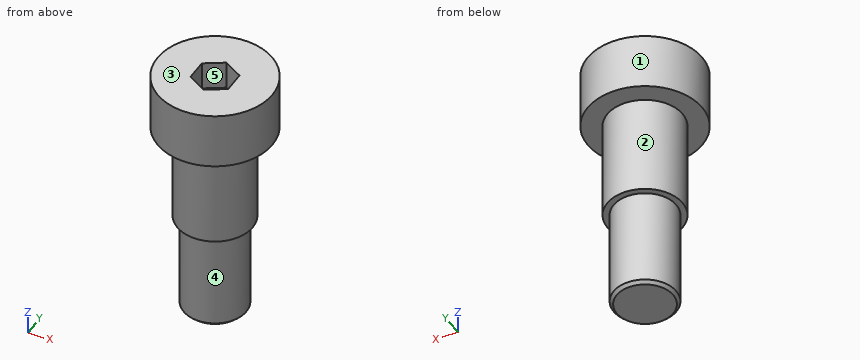
Solid Edge part; units mm, degrees
sketch "Sketch1" plane through (0, 0, 0) normal (0, 0, 1) x (1, 0, 0)
  circle A0 centre (0, 0) radius 9.135
extrude "Protrusion1" add sketch "Sketch1" along normal blind 9
sketch "Sketch2" plane through (0, 0, 9) normal (0, 0, 1) x (1, 0, 0)
  line L0 (0, -3.4641) -> (-3, -1.7321)
  line L1 (-3, -1.7321) -> (-3, 1.7321)
  line L2 (-3, 1.7321) -> (0, 3.4641)
  line L3 (0, 3.4641) -> (3, 1.7321)
  line L4 (3, 1.7321) -> (3, -1.7321)
  line L5 (3, -1.7321) -> (0, -3.4641)
extrude "Cutout1" cut sketch "Sketch2" against normal blind 4.5
sketch "Sketch3" plane through (0, 0, 0) normal (0, 0, -1) x (0, 1, 0)
  circle A0 centre (0, 0) radius 6
extrude "Protrusion2" add sketch "Sketch3" along normal blind 16
sketch "Sketch4" plane through (0, 0, -16) normal (0, 0, -1) x (0, 1, 0)
  circle A0 centre (0, 0) radius 5
extrude "Protrusion3" add sketch "Sketch4" along normal blind 16
chamfer "Chamfer1" distance 0.5 angle 45 1 edges at (0, -5, -32)
properties part number "221437"
Work out the finished part from the listing and answer in its coordinate system (mm). Face numbers are marked on the shaded views. A direction names the side the tool comes from. Round coordinates to 2 decimals unless told otherwise and drop trailing zeros. Loops run counter-clockwise (first coordinate to the right, second up) from the corner with the lowest first, then second, coordinate; pieces in that order, holes last.
(1) The mould has two halves that part along Y. Classify the marked faces 3, 4 and 5: pulls with the +Y half, pulls with the -Y half, needs draft (parallel to the pull), parting line crosses it, or undercut.
Computed values:
face 3: needs draft
face 4: parting line crosses it
face 5: undercut
(2) The part is cut by section B-B, the plane x = -5.5. Give the vertices of the cut face in (y, z).
Computed values:
outline: (-7.29, 0) - (-2.4, 0) - (-2.4, -16) - (2.4, -16) - (2.4, 0) - (7.29, 0) - (7.29, 9) - (-7.29, 9) - close
(3) The part is cut by section A-A, the plane y = 0. Give the vertices of the cut face in (x, z) (3 decimals).
Computed values:
outline: (-9.135, 0) - (-6, 0) - (-6, -16) - (-5, -16) - (-5, -31.5) - (-4.5, -32) - (4.5, -32) - (5, -31.5) - (5, -16) - (6, -16) - (6, 0) - (9.135, 0) - (9.135, 9) - (3, 9) - (3, 4.5) - (-3, 4.5) - (-3, 9) - (-9.135, 9) - close
(4) Find the intervals of material crossed by L1, parallel to Z at x = 3.75, y = 6.5; L2, parallel to Z at x = -0.25, y = -2.75; L3, parallel to X at y = -1.5, z = 5, in increasing order.
Computed values:
L1: z = 0 to 9
L2: z = -32 to 4.5
L3: x = -9.01 to -3, 3 to 9.01
(5) The part is cut by section C-C, the plane z = -15. Give the vertices of the cut face in (x, y), and give its area (3 significant figures).
Computed values:
outline: circle Ø12 at (0, 0)
area: 113 mm2
(6) The part is cut by section D-D, the plane z = 1. Give the vertices of the cut face in (x, y) (3 decimals), and give its area (3 significant figures).
Computed values:
outline: circle Ø18.27 at (0, 0)
area: 262 mm2
(7) Each of these flat-tipped pins is pushed along its axis until it touches: P1, Ø4, axis at y = -1, z = 6.5, coming from the -X side (3 decimals); P2, Ø5, axis at x = -3, z = -5, coming from the -Y side; P3, Ø4, axis at y = 2.5, z = -1, coming from the +X side; P4, Ø4, axis at y = 2, z = -11, coming from the +X side. Where does it stop, or does it pass through?
Computed values:
P1: stops at x = -9.135
P2: stops at y = -5.98
P3: stops at x = 9.1
P4: stops at x = 6
(8) For the marked faces 1 and 2, determine the directions among +Z, -Z, +X, -X, +Y, -Y from which every point of the face is accessible in a straight line to the end or side of a thin tool.
Computed values:
face 1: +Z, -Z
face 2: -Z
